Geometry check sheet. Reference: drawing and pictorial views, mm from the part's lowest x, y, z. A direction names the side the tool comes from. Coordinates: 2 decimals unless noted, no trailing zeros. Write each loop counter-clockwise with the first axis right and the second up, starting at its lowest first coordinate (ties: lowest second). Pieces come first, ordered by that corner, then holes. Notation, with made-up numbers: M 0,-2.75 L 40,-2.75 A19 ccw 40,13.25 Z; hole C 41,-23.5 d4. An arc over 180 degrees is marked long. One line per item, written item: value.
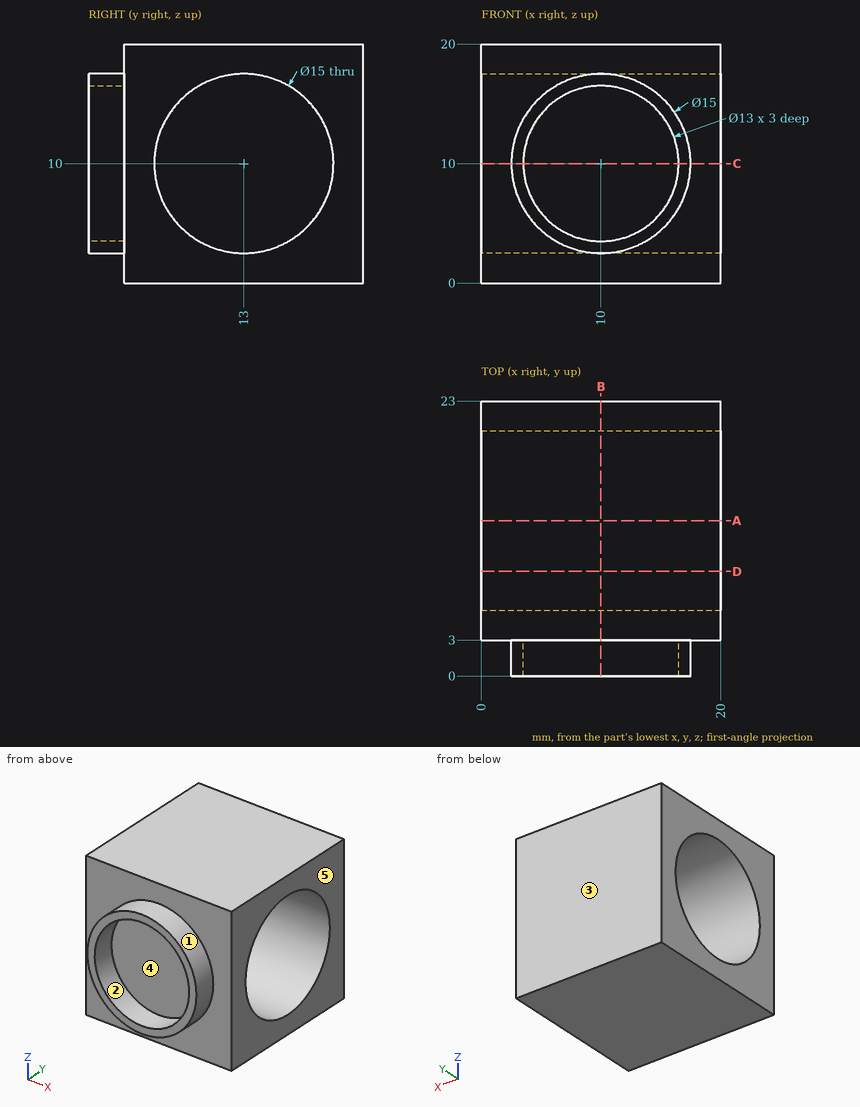
Item 1: Go/stop test with a flat-tipped pin: P1, Ø4, axis at x = 11.5, z = 11.5, coming from the -Y side. Record where the tip stops, or that it passes through.
The answers:
P1: stops at y = 3
Item 2: Access from +Z, -Z, +X, -X, +Y, -Y to the whole of each face (thin tool, end or side, straight path). Record for the marked faces 4 and 5.
The answers:
face 4: -Y
face 5: +Z, -Z, +X, +Y, -Y
Item 3: Cross-section at B-B, the plane x = 10. Enter the section's corners in (y, z), and give its area (3 significant figures).
The answers:
outline: M 0,2.5 L 3,2.5 L 3,0 L 23,0 L 23,20 L 3,20 L 3,17.5 L 0,17.5 L 0,16.5 L 3,16.5 L 3,3.5 L 0,3.5 Z; hole C 13,10 d15
area: 229 mm²
Item 4: Cross-section at C-C, the plane z = 10. Enter the section's corners in (x, y), and give its area (3 significant figures).
The answers:
outline: M 0,3 L 2.5,3 L 2.5,0 L 3.5,0 L 3.5,3 L 16.5,3 L 16.5,0 L 17.5,0 L 17.5,3 L 20,3 L 20,5.5 L 0,5.5 Z; M 0,20.5 L 20,20.5 L 20,23 L 0,23 Z
area: 106 mm²
Item 5: Scan lines: line 1 (X direction, y = 2.15, z = 10); line 2 (Y direction, x = 4.5, z = 10); line 3 (Z direction, x = 5.5, y = 16.75). Record each from-to range of solid material in increasing order.
The answers:
line 1: x = 2.5 to 3.5, 16.5 to 17.5
line 2: y = 3 to 5.5, 20.5 to 23
line 3: z = 0 to 3.5, 16.5 to 20
Item 6: Cross-section at D-D, the plane y = 8.75. Enter the section's corners in (x, z).
The answers:
outline: M 0,0 L 20,0 L 20,3.82 L 0,3.82 Z; M 0,16.18 L 20,16.18 L 20,20 L 0,20 Z
Item 7: Cross-section at A-A, the plane y = 13. Enter the section's corners in (x, z).
The answers:
outline: M 0,0 L 20,0 L 20,2.5 L 0,2.5 Z; M 0,17.5 L 20,17.5 L 20,20 L 0,20 Z
Item 8: Draft check along Z on the marked faces 1, 2 and 3. Enter one of: released by +Z, released by -Z, zero draft, split by the parting line, or undercut.
The answers:
face 1: split by the parting line
face 2: undercut
face 3: zero draft
